Model file for the job. Use its own axes, mm. A direction names the side the tool comes from. Coordinates: 2 decimals unless noted, no trailing zeros. Write each loop counter-clockwise with the first axis right and the second up, starting at its lowest first coordinate (ties: lowest second). Pieces come first, ordered by that corner, then holes. Notation, with made-up numbers: (52, 7.5) -> (73, 7.5) arc R32 cw to (73, 38.5) -> close; hole circle Ø7 at (-17.5, 88). An arc over 180 degrees is marked (long way). Answer as a JSON object with one key per item and string values. Group by question number.
from build123d import *

# Parameters (mm, degrees)
EXTRUDE_1_DEPTH     = 3
FILLET_1_R          = 5
CUT_EXTRUDE_1_REACH = 105.799
SKETCH_2_R          = 37.5


with BuildPart() as part:
    # 草圖1 → 填料-伸長1 (new body)
    with BuildSketch(Plane.XY):
        with BuildLine():
            Line((-47.5, 67), (-47.5, -67))
            Line((-47.5, -67), (-55.5, -67))
            ThreePointArc((-55.5, -67), (-59.5, -71), (-55.5, -75))
            Line((-55.5, -75), (-47.5, -75))
            Line((-47.5, -75), (-47.5, -85))
            Line((-47.5, -85), (47.5, -85))
            Line((47.5, -85), (47.5, -75))
            Line((47.5, -75), (55.5, -75))
            ThreePointArc((55.5, -75), (59.5, -71), (55.5, -67))
            Line((55.5, -67), (47.5, -67))
            Line((47.5, -67), (47.5, 67))
            Line((47.5, 67), (55.5, 67))
            ThreePointArc((55.5, 67), (59.5, 71), (55.5, 75))
            Line((55.5, 75), (47.5, 75))
            Line((47.5, 75), (47.5, 85))
            Line((47.5, 85), (-47.5, 85))
            Line((-47.5, 85), (-47.5, 75))
            Line((-47.5, 75), (-55.5, 75))
            ThreePointArc((-55.5, 75), (-59.5, 71), (-55.5, 67))
            Line((-55.5, 67), (-47.5, 67))
        make_face()
    extrude(amount=EXTRUDE_1_DEPTH)

    # 圓角1
    fillet_1_edges = [part.edges().sort_by_distance(p)[0] for p in [
        (-47.5, 85, 1.5),
        (47.5, 85, 1.5),
        (47.5, 75, 1.5),
        (47.5, 67, 1.5),
        (47.5, -67, 1.5),
        (47.5, -75, 1.5),
        (47.5, -85, 1.5),
        (-47.5, -85, 1.5),
        (-47.5, -75, 1.5),
        (-47.5, -67, 1.5),
        (-47.5, 67, 1.5),
        (-47.5, 75, 1.5),
    ]]
    fillet(fillet_1_edges, radius=FILLET_1_R - 0.0001)  # a hair under: the kernel refuses the full size

    # 草圖2 → 除料-伸長1 (cut, up to next)
    with BuildSketch(Plane.XY.offset(3), mode=Mode.PRIVATE) as cut_extrude_1_sk1:
        with Locations((0, 42.5)):
            Circle(SKETCH_2_R)
    cut_extrude_1_tool1 = extrude(cut_extrude_1_sk1.sketch, amount=-CUT_EXTRUDE_1_REACH, mode=Mode.PRIVATE) & part.part
    # 草圖2 → 除料-伸長1 (cut, up to next)
    with BuildSketch(Plane.XY.offset(3), mode=Mode.PRIVATE) as cut_extrude_1_sk2:
        with Locations((0, -42.5)):
            Circle(SKETCH_2_R)
    cut_extrude_1_tool2 = extrude(cut_extrude_1_sk2.sketch, amount=-CUT_EXTRUDE_1_REACH, mode=Mode.PRIVATE) & part.part
    add(cut_extrude_1_tool1.solids().sort_by_distance((0, 42.5, 3))[0], mode=Mode.SUBTRACT)
    add(cut_extrude_1_tool2.solids().sort_by_distance((0, -42.5, 3))[0], mode=Mode.SUBTRACT)


solid = part.part
(1) Pin check, flat tips, straight feed: pin 1 (0.9 mm diameter, centred on y = -19.5, z = 1.5, fed in from +X); pin 2 (1.5 mm diameter, centred on x = -53.5, z = 2, fed in from -Y); pin 3 (0.9 mm diameter, centred on x = 53.5, z = 2, fed in from +Y). Stop position of each tip, or through.
(2) Cut at B-B on x = 0. List the corners of the cut face in (y, z), plus the area to 3 significant figures.
(3) Cut at C-C on z = 1.75. Give the number of separate pieces and of enclosed holes in the cut face, plus the area to 3 significant figures.
(4) Wall check: probe 1 along Y at (x, z) = (0, 2.2); probe 2 along Y at (x, z) = (-27, 0.4); probe 3 along Y at (x, z) = (-53.5, 1). Give the ranges that are in metal, low to high.
(5) Cut at D-D on y = 18. List the corners of the cut face in (x, z), plus the area to 3 significant figures.
(6) Cut at A-A on y = -42.5. List the corners of the cut face in (x, z).
(7) Pull direction Y, two halves, no side cores. Call faces 1 (the face through (48.93, -76.5, 1.52)), 2 (the face through (-8.13, 5.89, 1.52)), 3 (the face through (-48.93, 65.5, 1.52)), 4 (the face through (46.07, 83.5, 1.52)): released by +Y, released by -Y, zero draft, split by the parting line, or undercut.
(8) 3-axis set-ups, long thin cutter, end or side, ignore diameter. For faces 5 (the face through (-46, 83.57, 1.52)), 6 (the face through (48.93, 65.5, 1.52)), 7 (the face through (-48.93, -65.5, 1.52)): which of +Z, -Z, +X, -X, +Y, -Y reach the whole face in a straight line?
Results found:
{
 "1": {"pin 1": "stops at x = 47.5", "pin 2": "stops at y = -75", "pin 3": "stops at y = 75"},
 "2": {"outline": "(-85, 0) -> (-80, 0) -> (-80, 3) -> (-85, 3) -> close; (-5, 0) -> (5, 0) -> (5, 3) -> (-5, 3) -> close; (80, 0) -> (85, 0) -> (85, 3) -> (80, 3) -> close", "area": "60.0 mm²"},
 "3": {"separate pieces": "1", "enclosed holes": "2", "area": "7,690 mm²"},
 "4": {"probe 1": "y = -85 to -80, -5 to 5, 80 to 85", "probe 2": "y = -85 to -68.52, -16.48 to 16.48, 68.52 to 85", "probe 3": "y = -75 to -67, 67 to 75"},
 "5": {"outline": "(-47.5, 0) -> (-28.39, 0) -> (-28.39, 3) -> (-47.5, 3) -> close; (28.39, 0) -> (47.5, 0) -> (47.5, 3) -> (28.39, 3) -> close", "area": "115 mm²"},
 "6": {"outline": "(-47.5, 0) -> (-37.5, 0) -> (-37.5, 3) -> (-47.5, 3) -> close; (37.5, 0) -> (47.5, 0) -> (47.5, 3) -> (37.5, 3) -> close"},
 "7": {"face 1": "released by -Y", "face 2": "undercut", "face 3": "undercut", "face 4": "released by +Y"},
 "8": {"face 5": "+Z, -Z, -X, +Y", "face 6": "+Z, -Z, +X", "face 7": "+Z, -Z, -X"}
}
